```python
from build123d import *

# Parameters (mm, degrees)
BOSS_EXTRUDE1_DEPTH     = 11.5
SKETCH4_R               = 3.075
CUT_EXTRUDE1_DEPTH      = 6
CUT_EXTRUDE6_DEPTH      = 4.6
CUT_EXTRUDE3_DEPTH      = 108.055479192
CUT_EXTRUDE3_DEPTH_BACK = 3.7
SKETCH24_W              = 82.375
SKETCH24_H              = 54
SKETCH25_R              = 1.35
CUT_EXTRUDE4_DEPTH      = 5
CHAMFER4_SIZE           = 0.5
FILLET1_R               = 2
BOSS_EXTRUDE2_DEPTH     = 0.8
CHAMFER5_SIZE           = 0.75


with BuildPart() as part:
    # Sketch1 → Boss-Extrude1 (new body)
    with BuildSketch(Plane(origin=(0, 0, 0), x_dir=(1, 0, 0), z_dir=(0, 1, 0))):
        with BuildLine():
            Line((-67.875, 67.5), (-67.875, -67.5))
            Line((-67.875, -67.5), (-67.875, -80.5))
            ThreePointArc((-67.875, -80.5), (-67.289213562, -81.914213562), (-65.875, -82.5))
            Line((-65.875, -82.5), (65.875, -82.5))
            ThreePointArc((65.875, -82.5), (67.289213562, -81.914213562), (67.875, -80.5))
            Line((67.875, -80.5), (67.875, -67.5))
            Line((67.875, -67.5), (67.875, 67.5))
            Line((67.875, 67.5), (67.875, 80.5))
            ThreePointArc((67.875, 80.5), (67.289213562, 81.914213562), (65.875, 82.5))
            Line((65.875, 82.5), (-65.875, 82.5))
            ThreePointArc((-65.875, 82.5), (-67.289213562, 81.914213562), (-67.875, 80.5))
            Line((-67.875, 80.5), (-67.875, 67.5))
        make_face()
    extrude(amount=BOSS_EXTRUDE1_DEPTH)

    # Sketch4 → Cut-Extrude1 (cut)
    with BuildSketch(Plane(origin=(0, 11.5, 0), x_dir=(1, 0, 0), z_dir=(0, 1, 0))):
        with Locations(Location((-59.875, -76, 0), (0, 0, 270))):
            Circle(SKETCH4_R)
        with Locations(Location((59.875, -76, 0), (0, 0, 270))):
            Circle(SKETCH4_R)
        with Locations(Location((59.875, 76, 0), (0, 0, 270))):
            Circle(SKETCH4_R)
        with Locations(Location((-59.875, 76, 0), (0, 0, 270))):
            Circle(SKETCH4_R)
    extrude(amount=-CUT_EXTRUDE1_DEPTH, mode=Mode.SUBTRACT)

    # Sketch21 → Cut-Extrude6 (cut)
    with BuildSketch(Plane(origin=(0, 11.5, 0), x_dir=(1, 0, 0), z_dir=(0, 1, 0))):
        Polygon((67.875, 31), (67.875, -31), (67.875, -31.25), (42.603553391, -31.25), (38.603553391, -35.25), (-22.75, -35.25), (-22.75, 35.25), (38.603553391, 35.25), (42.603553391, 31.25), (67.875, 31.25), align=None)
    extrude(amount=-CUT_EXTRUDE6_DEPTH, mode=Mode.SUBTRACT)

    # Sketch24 → Cut-Extrude3 (cut, two sides: drawn at the far end of the back side and taken through both)
    with BuildSketch(Plane(origin=(0, 6.9, 0), x_dir=(1, 0, 0), z_dir=(0, 1, 0)).offset(-CUT_EXTRUDE3_DEPTH_BACK)):
        with Locations((26.6875, 0)):
            Rectangle(SKETCH24_W, SKETCH24_H)
    extrude(amount=CUT_EXTRUDE3_DEPTH + CUT_EXTRUDE3_DEPTH_BACK, mode=Mode.SUBTRACT)

    # Sketch25 → Cut-Extrude4 (cut)
    with BuildSketch(Plane(origin=(0, 6.9, 0), x_dir=(1, 0, 0), z_dir=(0, 1, 0))):
        with Locations(Location((33.5, 30, 0), (0, 0, 270))):
            Circle(SKETCH25_R)
        with Locations(Location((-17.5, 30, 0), (0, 0, 270))):
            Circle(SKETCH25_R)
        with Locations(Location((33.5, -30, 0), (0, 0, 270))):
            Circle(SKETCH25_R)
        with Locations(Location((-17.5, -30, 0), (0, 0, 270))):
            Circle(SKETCH25_R)
    extrude(amount=-CUT_EXTRUDE4_DEPTH, mode=Mode.SUBTRACT)

    # Chamfer4
    chamfer4_edges = [part.edges().sort_by_distance(p)[0] for p in [
        (-17.5, 6.9, -31.35),
        (33.5, 6.9, 28.65),
        (-17.5, 6.9, 28.65),
        (33.5, 6.9, -31.35),
    ]]
    chamfer(chamfer4_edges, length=CHAMFER4_SIZE)

    # Fillet1
    fillet1_edges = [part.edges().sort_by_distance(p)[0] for p in [
        (26.6875, 3.2, -27),
        (-14.5, 5.05, -27),
        (-14.5, 3.2, 0),
        (-14.5, 5.05, 27),
        (26.6875, 3.2, 27),
    ]]
    fillet(fillet1_edges, radius=FILLET1_R)

    # Sketch26 → Boss-Extrude2 (add)
    with BuildSketch(Plane(origin=(0, 6.9, 0), x_dir=(1, 0, 0), z_dir=(0, 1, 0))):
        Polygon((38.603553391, 35.25), (38.603553391, 27), (67.875, 27), (67.875, 31.25), (42.603553391, 31.25), align=None)
        Polygon((42.603553391, -31.25), (38.603553391, -35.25), (38.603553391, -27), (67.875, -27), (67.875, -31.25), align=None)
    extrude(amount=BOSS_EXTRUDE2_DEPTH)

    # Chamfer5
    chamfer5_edges = [part.edges().sort_by_distance(p)[0] for p in [
        (-59.875, 11.5, -79.075),
        (59.875, 11.5, -79.075),
        (59.875, 11.5, 72.925),
        (-59.875, 11.5, 72.925),
    ]]
    chamfer(chamfer5_edges, length=CHAMFER5_SIZE)


solid = part.part
```
Check sheet for the modelled part. Datum: model origin and axes. Units: mm. A direction names the side the tool comes from. Round coordinates to 2 decimals unless told otherwise and drop trailing zeros. Loops run counter-clockwise (first coordinate to the right, second up) from the corner with the lowest first, then second, coordinate; pieces in that order, holes last. Notation, with made-up numbers: (1.5, -14) - (33.5, -14) arc R11 ccw to (33.5, -1) - close; hole circle Ø2 at (56, 82.5). An arc over 180 degrees is marked (long way). Answer as a JSON object with one key per item and string values. Group by question number.
Q1. Mould release check, pull along X, two halves, no side actions. Record for faces 4 (the face through (60, 5.5, 76)), 5 (the face through (-1, 6, 82.5)): released by +X, released by -X, zero draft, split by the parting line, or undercut.
Q2. Gauge pin test, flat ends, axial feed: P1, Ø2, axis at x = -17.5, z = -30, coming from the +Y side; P2, Ø1.8, axis at x = 59.5, z = 77, coming from the +Y side; P3, Ø2, axis at x = -18, z = 30, coming from the +Y side. Record the tip position at first contact, or that the pin passes through.
Q3. Set-up check for faces 1 (the face through (60, 5.5, -76)), 2 (the face through (-1, 0, -1)), 3 (the face through (55, 10, -31.25)): record each of +Z, -Z, +X, -X, +Y, -Y from which the full face is reachable in a straight line by a thin tool's end or side.
Q4. Scan lines: line 1 along X through (y, z) = (3.7, 30) (3 decimals); line 2 along X through (y, z) = (7.15, -76) (3 decimals); line 3 along Z through (x, y) = (43, 9). Record each from-to range of solid material in increasing order. Write a range as [from, to].
Q5. Sectioned sample at B-B, the plane x = 1. Enter the section's corners in (y, z).
Q6. Sectioned sample at C-C, the plane z = 76. Enter the section's corners in (x, y) (3 decimals).
Q7. Sectioned sample at A-A, the plane z = 21. Enter the section's corners in (x, y) (3 decimals).
Solution:
{
 "1": {"face 4": "undercut", "face 5": "zero draft"},
 "2": {"P1": "stops at y = 1.9", "P2": "stops at y = 5.5", "P3": "stops at y = 6.55"},
 "3": {"face 1": "+Y", "face 2": "+Z, -Z, +X, -X, -Y", "face 3": "+X, +Y"},
 "4": {"line 1": "x = [-67.875, -18.85], [-16.15, 32.15], [34.85, 67.875]", "line 2": "x = [-67.875, -62.95], [-56.8, 56.8], [62.95, 67.875]", "line 3": "z = [-82.5, -31.25], [31.25, 82.5]"},
 "5": {"outline": "(0, -82.5) - (11.5, -82.5) - (11.5, -35.25) - (6.9, -35.25) - (6.9, -27) - (5.2, -27) arc R2 cw to (3.2, -25) - (3.2, 25) arc R2 cw to (5.2, 27) - (6.9, 27) - (6.9, 35.25) - (11.5, 35.25) - (11.5, 82.5) - (0, 82.5) - close"},
 "6": {"outline": "(-67.875, 0) - (67.875, 0) - (67.875, 11.5) - (63.7, 11.5) - (62.95, 10.75) - (62.95, 5.5) - (56.8, 5.5) - (56.8, 10.75) - (56.05, 11.5) - (-56.05, 11.5) - (-56.8, 10.75) - (-56.8, 5.5) - (-62.95, 5.5) - (-62.95, 10.75) - (-63.7, 11.5) - (-67.875, 11.5) - close"},
 "7": {"outline": "(-67.875, 0) - (67.875, 0) - (67.875, 3.2) - (-12.5, 3.2) arc R2 cw to (-14.5, 5.2) - (-14.5, 6.9) - (-22.75, 6.9) - (-22.75, 11.5) - (-67.875, 11.5) - close"}
}
